Can you work these out from the model? Positions are in its coordinate system, mm. Give positions to 0.01 mm unless a question says otherwise; leave off trailing zeros. Order: outer loops, then holes, each group sorted by start corner. A loop starts at its lowest first (then second) coordinate and runs counter-clockwise, first axis right, second up. Notation, with made-up numbers: (29, -31.5) - (75, -31.5) arc R27 ccw to (75, -13.5) - close; hole circle Ø1 at (18, 79). An arc over 180 degrees is marked (long way). Return JSON: item names as keys, results as strings.
```python
from build123d import *

# Parameters (mm, degrees)
BOSS_EXTRUDE1_DEPTH        = 5
FILLET1_R                  = 1
CHAMFER2_SIZE              = 1
M10X1_25_TAPPED_HOLE1_D    = 8.8
F_10_0_10_DIAMETER_HOLE1_D = 10
CHAMFER3_SIZE              = 0.5


with BuildPart() as part:
    # Sketch2 → Boss-Extrude1 (new, symmetric)
    with BuildSketch(Plane(origin=(0, 0, 0), x_dir=(1, 0, 0), z_dir=(0, 1, 0))):
        with BuildLine():
            Line((49, 25), (-49, 25))
            ThreePointArc((-49, 25), (-49.707106781, 24.707106781), (-50, 24))
            Line((-50, 24), (-50, -24))
            ThreePointArc((-50, -24), (-49.707106781, -24.707106781), (-49, -25))
            Line((-49, -25), (49, -25))
            ThreePointArc((49, -25), (49.707106781, -24.707106781), (50, -24))
            Line((50, -24), (50, 24))
            ThreePointArc((50, 24), (49.707106781, 24.707106781), (49, 25))
        make_face()
    extrude(amount=BOSS_EXTRUDE1_DEPTH, both=True)

    # Fillet1
    fillet1_edges = [part.edges().sort_by_distance(p)[0] for p in [
        (-49.707106781, 5, 24.707106781),
        (0, 5, 25),
        (49.707106781, 5, 24.707106781),
        (50, 5, 0),
        (49.707106781, 5, -24.707106781),
        (0, 5, -25),
        (-49.707106781, 5, -24.707106781),
        (-50, 5, 0),
    ]]
    fillet(fillet1_edges, radius=FILLET1_R)

    # Chamfer2
    chamfer2_edges = [part.edges().sort_by_distance(p)[0] for p in [
        (0, -5, 25),
        (-49.707106781, -5, 24.707106781),
        (-50, -5, 0),
        (-49.707106781, -5, -24.707106781),
        (0, -5, -25),
        (49.707106781, -5, -24.707106781),
        (50, -5, 0),
        (49.707106781, -5, 24.707106781),
    ]]
    chamfer(chamfer2_edges, length=CHAMFER2_SIZE)

    # M10x1.25 Tapped Hole1 (through all)
    with Locations(Plane(origin=(-30, 5, -12.5), x_dir=(0, 0, 1), z_dir=(0, 1, 0))):
        with Locations((0, 0), (25, 0)):
            Hole(M10X1_25_TAPPED_HOLE1_D / 2)

    # 10.0 _10_ Diameter Hole1 (through all)
    with Locations(Plane(origin=(30, 5, -12.5), x_dir=(0, 0, 1), z_dir=(0, 1, 0))):
        with Locations((0, 0), (25, 0)):
            Hole(F_10_0_10_DIAMETER_HOLE1_D / 2)

    # Chamfer3
    chamfer3_edges = [part.edges().sort_by_distance(p)[0] for p in [
        (-30, 5, 16.9),
        (-30, 5, -8.1),
        (30, 5, 17.5),
        (30, 5, -7.5),
    ]]
    chamfer(chamfer3_edges, length=CHAMFER3_SIZE)


solid = part.part
```
1. For pin 1 Ø5.5 at (x, z) = (-30, -12.5) entering from +Y, with a flat end and sliding along its axis, tell me the tip position at first contact or that it passes through.
Checks:
{"pin 1": "through"}
2. Suppose I cut it at B-B (z = -12.5). List the corners of the cut face in (x, y) for me.
Checks:
{"outline": "(-50, -4) - (-49, -5) - (-34.4, -5) - (-34.4, 4.5) - (-34.9, 5) - (-49, 5) arc R1 ccw to (-50, 4) - close; (-25.6, -5) - (25, -5) - (25, 4.5) - (24.5, 5) - (-25.1, 5) - (-25.6, 4.5) - close; (35, -5) - (49, -5) - (50, -4) - (50, 4) arc R1 ccw to (49, 5) - (35.5, 5) - (35, 4.5) - close"}
3. Thinking about a two-plate mould opening in Z: for faces 1 (the face through (28.085, -0.317, -17.119)), 2 (the face through (-1, 0, 25)), 3 (the face through (-50, 0, 0)), which applies, +Z half, -Z half, draft (parallel to the pull), parting line (faces both ways), or undercut?
Checks:
{"face 1": "undercut", "face 2": "+Z half", "face 3": "draft"}
4. Suppose I cut it at C-C (y = -1.25). List the corners of the cut face in (x, z) for me, plus the area to 3 significant figures.
Checks:
{"outline": "(-50, -24) arc R1 ccw to (-49, -25) - (49, -25) arc R1 ccw to (50, -24) - (50, 24) arc R1 ccw to (49, 25) - (-49, 25) arc R1 ccw to (-50, 24) - close; hole circle Ø8.8 at (-30, -12.5); hole circle Ø8.8 at (-30, 12.5); hole circle Ø10 at (30, -12.5); hole circle Ø10 at (30, 12.5)", "area": "4,720 mm^2"}
5. Suppose I cut it at A-A (x = 30). List the corners of the cut face in (y, z) for me, plus the area to 3 significant figures.
Checks:
{"outline": "(-5, -24) - (-4, -25) - (4, -25) arc R1 ccw to (5, -24) - (5, -18) - (4.5, -17.5) - (-5, -17.5) - close; (-5, -7.5) - (4.5, -7.5) - (5, -7) - (5, 7) - (4.5, 7.5) - (-5, 7.5) - close; (-5, 17.5) - (4.5, 17.5) - (5, 18) - (5, 24) arc R1 ccw to (4, 25) - (-4, 25) - (-5, 24) - close", "area": "298 mm^2"}
6. If I drill on L1, parallel to X at y = 0.25, z = -12.5; L2, parallel to X at y = 3.75, z = 11; L3, parallel to Z at x = 26.5, y = -2.5, over which ranges is the centre line in solid material (lowest first)? Write a range as [from, to].
Checks:
{"L1": "[-50, -34.4], [-25.6, 25], [35, 50]", "L2": "[-50, -34.14], [-25.86, 25.23], [34.77, 50]", "L3": "[-25, -16.07], [-8.93, 8.93], [16.07, 25]"}
